```python
from build123d import *

# Parameters (mm, degrees)
F0_R     = 9.525
F1_DEPTH = 6.35
F2_SIZE  = 2.54


with BuildPart() as f1:
    # F0 (on Top) → F1 (new body)
    with BuildSketch(Plane.XY):
        Polygon((50.8, 101.6), (-50.8, 101.6), (-50.8, 0), (-50.8, -101.6), (50.8, -101.6), (50.8, 0), align=None)
        with Locations((-25.4, 76.2)):
            Circle(F0_R, mode=Mode.SUBTRACT)
        with Locations((25.4, 76.2)):
            Circle(F0_R, mode=Mode.SUBTRACT)
    extrude(amount=F1_DEPTH)

    # F2
    f2_edges = [f1.edges().sort_by_distance(p)[0] for p in [
        (-34.925, 76.2, 6.35),
        (15.875, 76.2, 6.35),
    ]]
    chamfer(f2_edges, length=F2_SIZE)


solid = f1.part
```
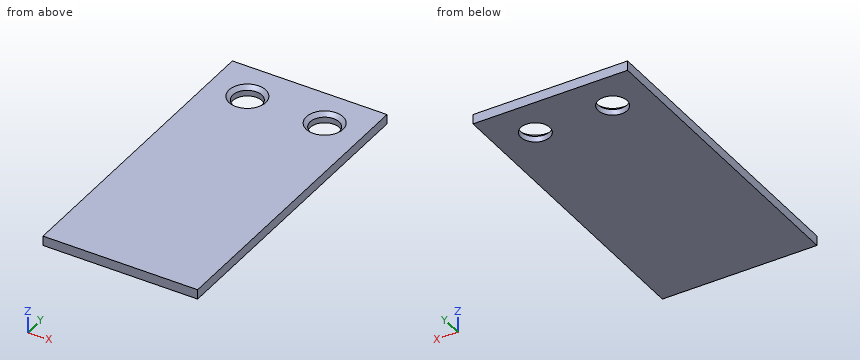
Can you work these out from the model? Positions are in its coordinate system, mm. Coordinates: 2 decimals unless noted, no trailing zeros. Loops run counter-clockwise (first coordinate to the right, second up) from the corner with the lowest first, then second, coordinate; pieces in that order, holes last.
1) I need wall thicknesses on probe 1 along Y at (x, z) = (-25.4, 1.2) (3 decimals); probe 2 along X at (y, z) = (83.5, 2.75); probe 3 along X at (y, z) = (67.5, 4). Which ranges of each line are inside material? Lowest first, please.
2) Imagine slicing it at A-A on y = 76.2. List the corners of the cut face in (x, z) for me (3 decimals), plus the area to 3 significant figures.
3) Imagine slicing it at C-C on x = -25.4. List the corners of the cut face in (y, z) for me (3 decimals).
4) Imagine slicing it at B-B on z = 1.75. List the corners of the cut face in (x, y) for me (3 decimals), plus the area to 3 significant figures.
5) For pin 1 (15 mm diameter, centred on x = 25.4, y = 76.2, fed in from +Z), with a flat end and sliding along its axis, tell me the tip position at first contact or that it passes through.
Completed:
1. probe 1: y = -101.6 to 66.675, 85.725 to 101.6
1. probe 2: x = -50.8 to -31.52, -19.28 to 19.28, 31.52 to 50.8
1. probe 3: x = -50.8 to -29.72, -21.08 to 21.08, 29.72 to 50.8
2. outline: (-50.8, 0) - (-34.925, 0) - (-34.925, 3.81) - (-37.465, 6.35) - (-50.8, 6.35) - close; (-15.875, 0) - (15.875, 0) - (15.875, 3.81) - (13.335, 6.35) - (-13.335, 6.35) - (-15.875, 3.81) - close; (34.925, 0) - (50.8, 0) - (50.8, 6.35) - (37.465, 6.35) - (34.925, 3.81) - close
2. area: 390 mm2
3. outline: (-101.6, 0) - (66.675, 0) - (66.675, 3.81) - (64.135, 6.35) - (-101.6, 6.35) - close; (85.725, 0) - (101.6, 0) - (101.6, 6.35) - (88.265, 6.35) - (85.725, 3.81) - close
4. outline: (-50.8, -101.6) - (50.8, -101.6) - (50.8, 101.6) - (-50.8, 101.6) - close; hole circle Ø19.05 at (-25.4, 76.2); hole circle Ø19.05 at (25.4, 76.2)
4. area: 20,100 mm2
5. pin 1: passes through
